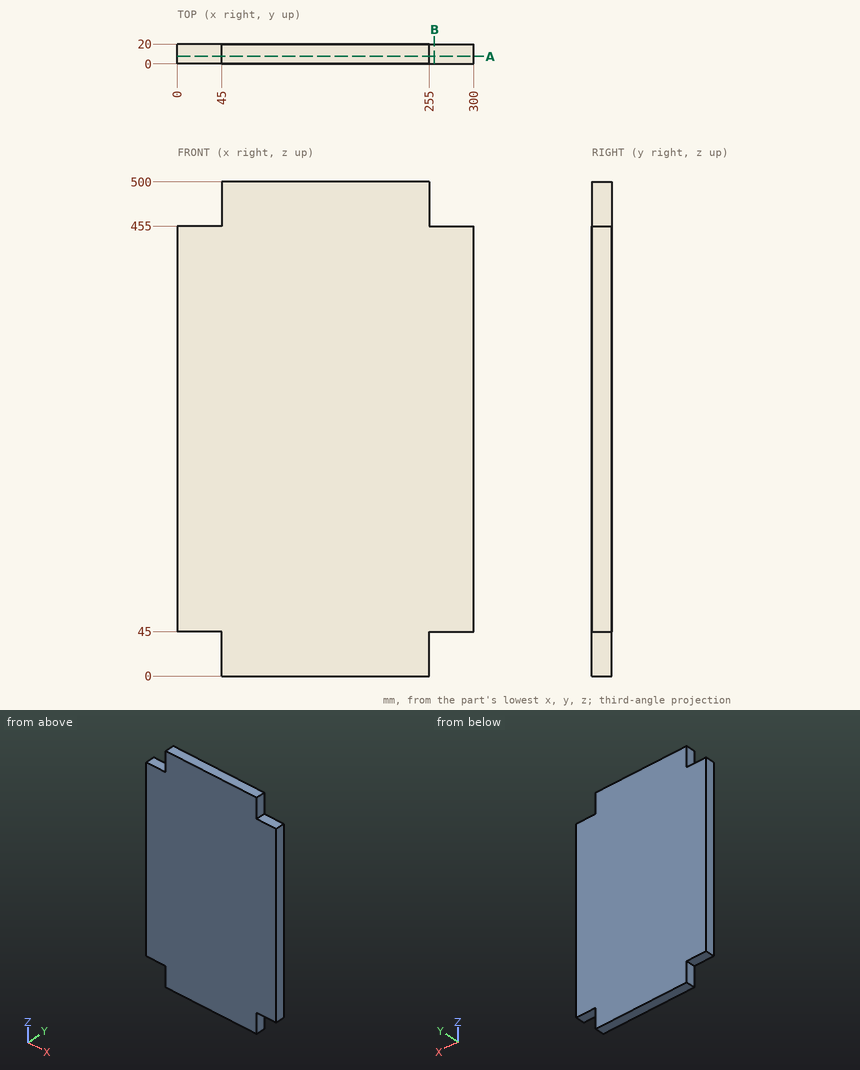
Input: dimensioned drawing with shaded views. Units: mm. Origin: part minimum x, y, z. Give positions to 0.01 mm unless a question says otherwise; leave off trailing zeros. Write each loop counter-clockwise with the first axis right and the second up, starting at its lowest first coordinate (ties: lowest second). Pieces come first, ordered by that corner, then holes. Notation, with made-up numbers: M 48,-9 L 105,-9 A25 ccw 105,18 Z; hole C -4,16 d6. An arc over 180 degrees is marked long. Return JSON: item names as keys, results as strings. Group by question number.
1) Cut plane B-B, the plane x = 260. Output: boundary loops of the cut face in (y, z).
2) Material intervals for line 1 along X through (y, z) = (7.5, 22.5); line 2 along Z through (x, y) = (27, 9), sorted ascending. Write a range as [from, to].
3) Cut plane A-A, the plane y = 7.5. Output: boundary loops of the cut face in (x, z), plus the area to 3 significant figures.
4) Pin query (flat end, axial travel): P1, Ø6, axis at x = 279, y = 12.5, coming from the -Z side; P2, Ø10, axis at y = 9.5, z = 33.5, coming from the +X side; P3, Ø10, axis at x = 272, y = 8.5, coming from the +Z side. Return the tip coordinate at first contact, or that it passes through.
Recorded:
{
 "1": {"outline": "M 0,45 L 20,45 L 20,455 L 0,455 Z"},
 "2": {"line 1": "x = [45, 255]", "line 2": "z = [45, 455]"},
 "3": {"outline": "M 0,45 L 45,45 L 45,0 L 255,0 L 255,45 L 300,45 L 300,455 L 255,455 L 255,500 L 45,500 L 45,455 L 0,455 Z", "area": "142,000 mm²"},
 "4": {"P1": "stops at z = 45", "P2": "stops at x = 255", "P3": "stops at z = 455"}
}
